```python
from build123d import *

# Parameters (mm, degrees)
EXTRUDE_1_DEPTH          = 4.45
EXTRUDE_1_DEPTH_BACK     = 4.45
SKETCH_1_W               = 10.5
SKETCH_1_H               = 14
SKETCH_1_W_2             = 7.5
SKETCH_1_H_2             = 9.5
SKETCH_2_R               = 2.5
CUT_EXTRUDE_1_DEPTH      = 5
CUT_EXTRUDE_2_DEPTH      = 13.480885385
CUT_EXTRUDE_2_DEPTH_BACK = 13.480885385
FILLET_1_R               = 1


with BuildPart() as part:
    # Sketch 1 → Extrude 1 (new, two sides: drawn at the far end of the back side and taken through both)
    with BuildSketch(Plane(origin=(0, 0, 0), x_dir=(0, 0, -1), z_dir=(1, 0, 0)).offset(-EXTRUDE_1_DEPTH_BACK)):
        Rectangle(SKETCH_1_W, SKETCH_1_H)
        with Locations((0, -0.75)):
            Rectangle(SKETCH_1_W_2, SKETCH_1_H_2, mode=Mode.SUBTRACT)
    extrude(amount=EXTRUDE_1_DEPTH + EXTRUDE_1_DEPTH_BACK)

    # Sketch 2 → Cut-Extrude 1 (cut)
    with BuildSketch(Plane(origin=(0, 7, 0), x_dir=(1, 0, 0), z_dir=(0, 1, 0))):
        with Locations(Location((0, 0, 0), (0, 0, 270))):
            Circle(SKETCH_2_R)
    extrude(amount=-CUT_EXTRUDE_1_DEPTH, mode=Mode.SUBTRACT)

    # Sketch 3 → Cut-Extrude 2 (cut, two sides: drawn at the far end of the back side and taken through both)
    with BuildSketch(Plane(origin=(4.45, 0, 0), x_dir=(0, 0, -1), z_dir=(1, 0, 0)).offset(-CUT_EXTRUDE_2_DEPTH_BACK)):
        Polygon((42.829414647, 29.662513803), (5.25, 6.470985869), (3.661056498, 5.490395087), (3.661056498, 5.306534315), (5.25, 5.306534315), (49.409476594, 5.306534315), (134.671683999, 28.341149153), (128.091622051, 52.697128641), align=None)
    extrude(amount=CUT_EXTRUDE_2_DEPTH + CUT_EXTRUDE_2_DEPTH_BACK, mode=Mode.SUBTRACT)

    # Fillet 1
    fillet_1_edges = [part.edges().sort_by_distance(p)[0] for p in [
        (0, 5.306534315, -5.25),
        (0, 7, 5.25),
        (0, -7, -5.25),
        (0, -7, 5.25),
    ]]
    fillet(fillet_1_edges, radius=FILLET_1_R)


solid = part.part
```
The listing builds one solid part. Answer for the finished solid, in the listing's coordinates (mm). A direction names the side the tool comes from. Coordinates: 2 decimals unless noted, no trailing zeros. Loops run counter-clockwise (first coordinate to the right, second up) from the corner with the lowest first, then second, coordinate; pieces in that order, holes last. Notation, with made-up numbers: M 35.25,10 L 65.25,10 A22 cw 65.25,44 Z; hole C 73,25.5 d4. An arc over 180 degrees is marked long. Answer as a JSON object with one key per item and string values. Group by question number.
Item 1: Consider L1, parallel to Z at x = -3.25, y = -3.75; L2, parallel to Y at x = -3.5, z = -0.75; L3, parallel to X at y = 5.75, z = 0. Determine where each line is inside the solid, lowest interval first.
Item 2: Section B-B (y = -5.25) is taken. Write down the section's boundary in (x, z), and give its area (3 significant figures).
Item 3: Section D-D (z = -3.5) is taken. Write down the section's boundary in (x, y), and give its area (4 significant figures).
Item 4: Which of the six approach directions +Z, -Z, +X, -X, +Y, -Y give full straight-line access (tool end or side, diameter ignored) to faces 5 (the face through (0, 4, 3)), 6 (the face through (-0.06, 5.99, -4.47)), 7 (the face through (0, -7, 0))?
Item 5: Determine the mould class of faces 1 (the face through (-2.44, 5.52, -0.54)), 2 (the face through (4.45, 5, 0)), 3 (the face through (0, -5.5, 0)), 4 (the face through (-4.45, 5, 0)) for opening direction X: +X half, -X half, draft (parallel to the pull), parting line (faces both ways), or undercut.
Item 6: Section C-C (x = -2) is taken. Write down the section's boundary in (y, z), and give its area (3 significant figures).
Item 7: This flat-tipped pin is pushed along its axis until it touches: P1, Ø3, axis at x = 0, z = 0, coming from the +Y side. Where does it stop, or does it pass through?
Item 8: Section A-A (z = 2) is taken. Write down the section's boundary in (x, y), and give its area (4 significant figures).
Solved:
{
 "1": {"L1": "z = -5.25 to -3.75, 3.75 to 5.25", "L2": "y = -7 to -5.5, 4 to 7", "L3": "x = -4.45 to -2.5, 2.5 to 4.45"},
 "2": {"outline": "M -4.45,-5.25 L 4.45,-5.25 L 4.45,-3.75 L -4.45,-3.75 Z; M -4.45,3.75 L 4.45,3.75 L 4.45,5.25 L -4.45,5.25 Z", "area": "26.7 mm2"},
 "3": {"outline": "M -4.45,-7 L 4.45,-7 L 4.45,-5.5 L -4.45,-5.5 Z; M -4.45,4 L 4.45,4 L 4.45,7 L -4.45,7 Z", "area": "40.05 mm2"},
 "4": {"face 5": "+X, -X", "face 6": "-Z, +X, -X", "face 7": "+Z, -Z, +X, -X, -Y"},
 "5": {"face 1": "undercut", "face 2": "+X half", "face 3": "draft", "face 4": "-X half"},
 "6": {"outline": "M -7,-4.25 A1 ccw -6,-5.25 L 4.31,-5.25 A1 ccw 5.31,-4.25 L 5.31,-3.66 L 5.49,-3.66 L 6.47,-5.25 L 7,-5.25 L 7,-1.5 L 4,-1.5 L 4,-3.75 L -5.5,-3.75 L -5.5,3.75 L 4,3.75 L 4,1.5 L 7,1.5 L 7,4.25 A1 ccw 6,5.25 L -6,5.25 A1 ccw -7,4.25 Z", "area": "64.8 mm2"},
 "7": {"P1": "stops at y = -5.5"},
 "8": {"outline": "M -4.45,-7 L 4.45,-7 L 4.45,-5.5 L -4.45,-5.5 Z; M -4.45,4 L -1.5,4 L -1.5,7 L -4.45,7 Z; M 1.5,4 L 4.45,4 L 4.45,7 L 1.5,7 Z", "area": "31.05 mm2"}
}
